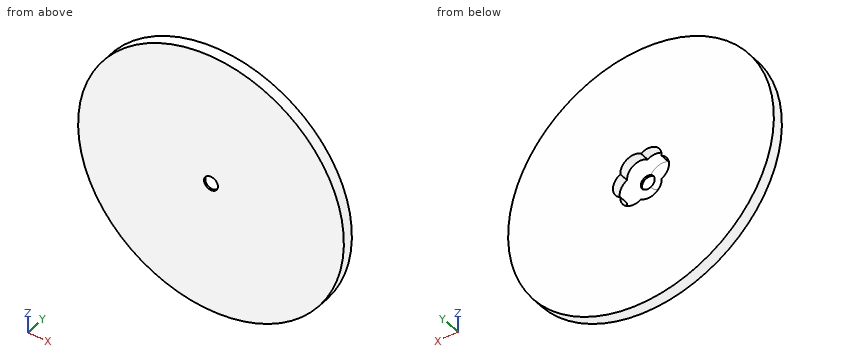
```python
from build123d import *

# Parameters (mm, degrees)
SKETCH1_R           = 95
BOSS_EXTRUDE1_DEPTH = 8
SKETCH2_R           = 5
CUT_EXTRUDE1_DEPTH  = 135.588261004
SKETCH3_R           = 9.498426828
CUT_EXTRUDE2_DEPTH  = 6.743986
CIRPATTERN1_START   = 1.25601425
CIRPATTERN1_DEPTH   = 6.74398575


# Read off the part's stored shape, not the designer's step: CirPattern1
with BuildPart() as part:
    # Sketch1 → Boss-Extrude1 (new body)
    with BuildSketch(Plane(origin=(0, 0, 0), x_dir=(1, 0, 0), z_dir=(0, 1, 0))):
        with Locations(Location((0, 0, 0), (0, 0, 270))):
            Circle(SKETCH1_R)
    extrude(amount=BOSS_EXTRUDE1_DEPTH)

    # Sketch2 → Cut-Extrude1 (cut, through all)
    with BuildSketch(Plane(origin=(0, 0, 0), x_dir=(1, 0, 0), z_dir=(0, 1, 0))):
        with Locations(Location((0, 0, 0), (0, 0, 270))):
            Circle(SKETCH2_R)
    extrude(amount=CUT_EXTRUDE1_DEPTH, mode=Mode.SUBTRACT)

    # Sketch3 → Cut-Extrude2 (cut)
    with BuildSketch(Plane(origin=(0, 8, 0), x_dir=(1, 0, 0), z_dir=(0, 1, 0))):
        with Locations((-10.59166458, 0)):
            Circle(SKETCH3_R)
    extrude(amount=-CUT_EXTRUDE2_DEPTH, mode=Mode.SUBTRACT)

    # CirPattern1 outline → CirPattern1 (cut)
    with BuildSketch(Plane(origin=(0, 0, 0), x_dir=(1, 0, 0), z_dir=(0, 1, 0)).offset(CIRPATTERN1_START)):
        with BuildLine():
            ThreePointArc((-2.216990824, -4.481623778), (-7.677514135, -9.040345092), (-14.772416271, -8.528858511))
            ThreePointArc((-14.772416271, -8.528858511), (-10.045045704, -17.398529523), (0, -17.057717022))
            ThreePointArc((0, -17.057717022), (10.045045704, -17.398529523), (14.772416271, -8.528858511))
            ThreePointArc((14.772416271, -8.528858511), (20.090091407, 0), (14.772416271, 8.528858511))
            ThreePointArc((14.772416271, 8.528858511), (10.045045704, 17.398529523), (0, 17.057717022))
            ThreePointArc((0, 17.057717022), (-10.045045704, 17.398529523), (-14.772416271, 8.528858511))
            ThreePointArc((-14.772416271, 8.528858511), (-7.677514135, 9.040345092), (-2.216990824, 4.481623778))
            ThreePointArc((-2.216990824, 4.481623778), (5, 0), (-2.216990824, -4.481623778))
        make_face()
    extrude(amount=CIRPATTERN1_DEPTH, mode=Mode.SUBTRACT)


solid = part.part
```
Part model, mm, in its own coordinate system. Round coordinates to 2 decimals unless told otherwise and drop trailing zeros. Loops run counter-clockwise (first coordinate to the right, second up) from the corner with the lowest first, then second, coordinate; pieces in that order, holes last. Notation, with made-up numbers: (30.25, 70) -> (38.25, 70) arc R20 ccw to (38.25, 88) -> close; hole circle Ø2 at (66.25, -28). An arc over 180 degrees is marked (long way). Use CSV: the item, a comma, the result in double quotes. Start each with the question number.
1) Wall check: L1, parallel to X at y = 0.75, z = 0; L2, parallel to Z at x = 11, y = 6.75; L3, parallel to X at y = 3.5, z = -15. Give the ranges that are in metal, low to high. Write a range as [from, to].
2) Cut at B-B, the plane y = 6.5. Write the cut outline in (x, z), plus the area to 3 significant figures.
3) Drop flat-ended pins along their axis: P1, Ø10.5, axis at x = 5.5, z = -1.5, coming from the +Y side; P2, Ø4, axis at x = 36, y = 2.5, coming from the -Z side; P3, Ø1.5, axis at x = -47.5, y = 4, coming from the -Z side. Give the stop position or say it passes through.
4) Cut at A-A, the plane z = 0. Write the cut outline in (x, y), plus the area to 3 significant figures.
5) Cut at D-D, the plane z = -25.5. Write the cut outline in (x, y), plus the area to 3 significant figures.
6) Cut at C-C, the plane x = 54. Write the cut outline in (y, z), plus the area to 3 significant figures.
Determined:
1,L1,"x = [-95, -5], [5, 95]"
1,L2,"z = [-94.36, -16.77], [16.77, 94.36]"
1,L3,"x = [-93.81, -12.8], [12.8, 93.81]"
2,outline,"circle Ø190 at (0, 0); hole (-14.77, -8.53) arc R9.5 ccw to (0, -17.06) arc R9.5 ccw to (14.77, -8.53) arc R9.5 ccw to (14.77, 8.53) arc R9.5 ccw to (0, 17.06) arc R9.5 ccw to (-14.77, 8.53) arc R9.5 ccw to start"
2,area,"27,200 mm2"
3,P1,"stops at y = 1.26"
3,P2,"stops at z = -88.71"
3,P3,"stops at z = -82.7"
4,outline,"(-95, 0) -> (-5, 0) -> (-5, 1.26) -> (-20.09, 1.26) -> (-20.09, 8) -> (-95, 8) -> close; (5, 0) -> (95, 0) -> (95, 8) -> (20.09, 8) -> (20.09, 1.26) -> (5, 1.26) -> close"
4,area,"1,240 mm2"
5,outline,"(-91.51, 0) -> (91.51, 0) -> (91.51, 8) -> (-91.51, 8) -> close"
5,area,"1,460 mm2"
6,outline,"(0, -78.16) -> (8, -78.16) -> (8, 78.16) -> (0, 78.16) -> close"
6,area,"1,250 mm2"
